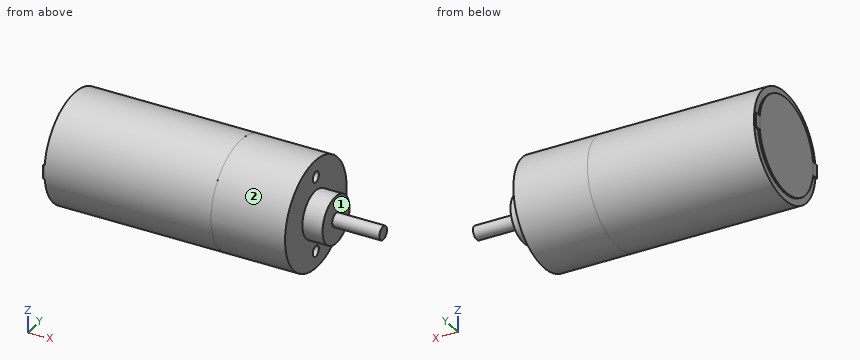
Autodesk Inventor part; units mm, degrees
ref_plane "YZ Plane" through (0, 0, 0) normal (1, 0, 0) x (0, 1, 0)
ref_plane "XZ Plane" through (0, 0, 0) normal (0, 1, 0) x (-1, 0, 0)
ref_plane "XY Plane" through (0, 0, 0) normal (0, 0, 1) x (1, 0, 0)
sketch "Sketch1" plane through (0, 0, 0) normal (1, 0, 0) x (0, 1, 0)
  circle A0 centre (0, 0) radius 8
  dimension "d0" = 16
sketch "Sketch1 outline for Extrusion1" plane through (0, 0, 0) normal (1, 0, 0) x (0, 1, 0)
  circle A0 centre (0, 0) radius 8
extrude "Extrusion1" add sketch "Sketch1 outline for Extrusion1" along normal blind 25
sketch "Sketch2" plane through (25, 0, 0) normal (1, 0, 0) x (0, 0, -1)
  circle A0 centre (0, 0) radius 8
  circle A1 centre (0, 0) radius 7.9985
  dimension "d20" = 15.997
sketch "Sketch2 outline for Extrusion2" plane through (25, 0, 0) normal (1, 0, 0) x (0, 0, -1)
  circle A0 centre (0, 0) radius 7.9985
extrude "Extrusion2" add sketch "Sketch2 outline for Extrusion2" along normal blind 11
sketch "Sketch3" plane through (36, 0, 0) normal (1, 0, 0) x (0, 0, -1)
  circle A0 centre (0, 0) radius 8 construction
  line L0 (-8, 0) -> (8, 0) construction
  circle A1 centre (0, 0) radius 5.5 construction
  point P0 (-5.5, 0)
  point P1 (5.5, 0)
  dimension "d6" = 11
hole "Hole1" at (36, 0, 5.5) at (36, 0, -5.5) direction (-1, 0, 0) diameter 1.567 depth 4
sketch "Sketch4" plane through (36, 0, 0) normal (1, 0, 0) x (0, 0, -1)
  circle A0 centre (-5.5, 0) radius 0.7835
  circle A1 centre (5.5, 0) radius 0.7835
  circle A2 centre (0, 0) radius 3.5
  dimension "d14" = 7
sketch "Sketch4 outline for Extrusion3" plane through (36, 0, 0) normal (1, 0, 0) x (0, 0, -1)
  circle A0 centre (0, 0) radius 3.5
extrude "Extrusion3" add sketch "Sketch4 outline for Extrusion3" along normal blind 3
sketch "Sketch5" plane through (39, 0, 0) normal (1, 0, 0) x (0, 0, -1)
  circle A0 centre (0, 0) radius 1
  dimension "d17" = 2
sketch "Sketch5 outline for Extrusion4" plane through (39, 0, 0) normal (1, 0, 0) x (0, 0, -1)
  circle A0 centre (0, 0) radius 1
extrude "Extrusion4" add sketch "Sketch5 outline for Extrusion4" along normal blind 7
sketch "Sketch6" plane through (0, 0, 0) normal (-1, 0, 0) x (0, 0, 1)
  circle A0 centre (0, 0) radius 7
  circle A1 centre (0, 0) radius 8
  line L0 (1, 6.928203) -> (-1, 6.928203)
  line L1 (-1, 6.928203) -> (-1, 7.928203)
  line L2 (-1, 7.928203) -> (1, 7.928203)
  line L3 (1, 7.928203) -> (1, 6.928203)
  line L4 (1, -6.928203) -> (-1, -6.928203)
  line L5 (-1, -6.928203) -> (-1, -7.928203)
  line L6 (-1, -7.928203) -> (1, -7.928203)
  line L7 (1, -7.928203) -> (1, -6.928203)
  dimension "d21" = 1
  dimension "d22" = 2
  dimension "d23" = 1
sketch "Sketch6 outline for Extrusion5" plane through (0, 0, 0) normal (-1, 0, 0) x (0, 0, 1)
  circle A0 centre (0, 0) radius 8
  arc A1 (-1, 6.928203) -> (-1, -6.928203) centre (0, 0) ccw
  line L0 (-1, -6.928203) -> (-1, -7.928203)
  line L1 (-1, -7.928203) -> (1, -7.928203)
  line L2 (1, -7.928203) -> (1, -6.928203)
  arc A2 (1, -6.928203) -> (1, 6.928203) centre (0, 0) ccw
  line L3 (1, 6.928203) -> (1, 7.928203)
  line L4 (1, 7.928203) -> (-1, 7.928203)
  line L5 (-1, 7.928203) -> (-1, 6.928203)
extrude "Extrusion5" cut sketch "Sketch6 outline for Extrusion5" against normal blind 0.25
sketch "Sketch6 outline for Extrusion6" plane through (0, 0, 0) normal (-1, 0, 0) x (0, 0, 1)
  arc A0 (1, -6.928203) -> (1, 6.928203) centre (0, 0) ccw
  line L0 (-1, -6.928203) -> (1, -6.928203)
  arc A1 (-1, 6.928203) -> (-1, -6.928203) centre (0, 0) ccw
  line L1 (1, 6.928203) -> (-1, 6.928203)
extrude "Extrusion6" cut sketch "Sketch6 outline for Extrusion6" against normal blind 0.01
properties part number "MotorNM" material "Steel, Galvanized"
Build history of the part. All positions in model axes, mm. Face numbers are marked on the shaded views. A direction names the side the tool comes from. Coordinates: 2 decimals unless noted, no trailing zeros. Write each loop counter-clockwise with the first axis right and the second up, starting at its lowest first coordinate (ties: lowest second). Pieces come first, ordered by that corner, then holes. Notation, with made-up numbers: (77.5, 66.25) -> (130.5, 66.25) arc R19 cw to (130.5, 97.25) -> close; hole circle Ø10 at (-29.5, -6). An arc over 180 degrees is marked (long way). Use CSV: the item, a comma, the result in double quotes. Start each with the question number.
Q1. Drill centre lines: probe 1 along X at (y, z) = (6, -0.5); probe 2 along X at (y, z) = (0.75, 3.25); probe 3 along Y at (x, z) = (34.2, -5.5). Where is each one in solid material? Low to high.
Q2. Cut at C-C, the plane x = 6. List the corners of the cut face in (y, z).
Q3. 3-axis set-ups, long thin cutter, end or side, ignore diameter. For the marked faces 1 and 2: which of +Z, -Z, +X, -X, +Y, -Y reach the whole face in a straight line?
Q4. Flat gauge pins, fed straight in: pin 1 Ø1 at (x, y) = (25, 4.5) entering from +Z; pin 2 Ø5 at (y, z) = (-2.5, -3.5) entering from +X; pin 3 Ø3 at (y, z) = (-5, 0.5) entering from -X. Where does each tip first touch, or does it go through?
Checked values:
1,probe 1,"x = 0.01 to 36"
1,probe 2,"x = 0.01 to 39"
1,probe 3,"y = -5.81 to -0.78, 0.78 to 5.81"
2,outline,"circle Ø16 at (0, 0)"
3,face 1,"+X"
3,face 2,"+X, -X"
4,pin 1,"stops at z = 6.93"
4,pin 2,"stops at x = 39"
4,pin 3,"stops at x = 0.01"
